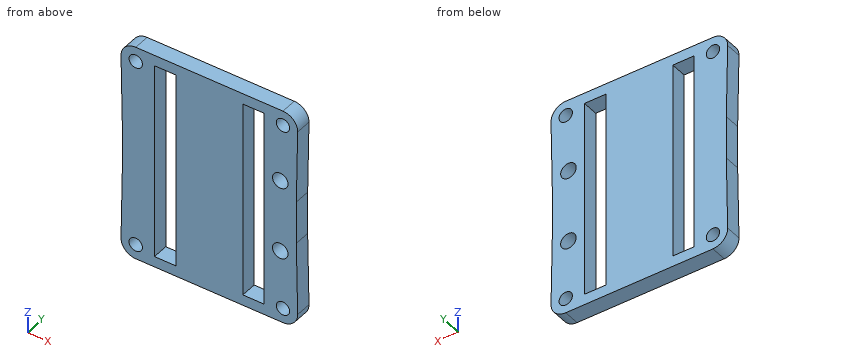
```python
from build123d import *

# Parameters (mm, degrees)
SKETCH1_R              = 1.25
SKETCH1_W              = 12.5
SKETCH1_H              = 37
BOSS_EXTRUDE1_DEPTH    = 3
M2_5_CLEARANCE_HOLE1_D = 2.9


with BuildPart() as part:
    # Sketch1 → Boss-Extrude1 (new body)
    with BuildSketch(Plane(origin=(0, 0, 0), x_dir=(1, 0, 0), z_dir=(0, 1, 0))):
        with BuildLine():
            Line((-16.25, -4), (-16.499543908, -17.699917074))
            ThreePointArc((-16.499543908, -17.699917074), (-15.712170743, -19.676755298), (-13.75, -20.5))
            Line((-13.75, -20.5), (13.75, -20.5))
            ThreePointArc((13.75, -20.5), (15.712170743, -19.676755298), (16.499543908, -17.699917074))
            Line((16.499543908, -17.699917074), (16.25, -4))
            Line((16.25, -4), (16.25, 0))
            Line((16.25, 0), (16.25, 4))
            Line((16.25, 4), (16.499543908, 17.699917074))
            ThreePointArc((16.499543908, 17.699917074), (15.712170743, 19.676755298), (13.75, 20.5))
            Line((13.75, 20.5), (-13.75, 20.5))
            ThreePointArc((-13.75, 20.5), (-15.712170743, 19.676755298), (-16.499543908, 17.699917074))
            Line((-16.499543908, 17.699917074), (-16.25, 4))
            Line((-16.25, 4), (-16.25, 0))
            Line((-16.25, 0), (-16.25, -4))
        make_face()
        with Locations((-13.75, -17.75)):
            Circle(SKETCH1_R, mode=Mode.SUBTRACT)
        with Locations((-13.75, 17.75)):
            Circle(SKETCH1_R, mode=Mode.SUBTRACT)
        with Locations((13.75, 17.75)):
            Circle(SKETCH1_R, mode=Mode.SUBTRACT)
        with Locations((13.75, -17.75)):
            Circle(SKETCH1_R, mode=Mode.SUBTRACT)
        Polygon((-6.25, 18.5), (-10.25, 18.5), (-10.25, -18.5), (-6.25, -18.5), (6.25, -18.5), (10.25, -18.5), (10.25, 18.5), (6.25, 18.5), align=None, mode=Mode.SUBTRACT)
        Rectangle(SKETCH1_W, SKETCH1_H)
    extrude(amount=BOSS_EXTRUDE1_DEPTH)

    # M2.5 Clearance Hole1 (through all)
    with Locations(Plane.XZ):
        with Locations((13.25, -6.8), (13.25, 6.8)):
            Hole(M2_5_CLEARANCE_HOLE1_D / 2)


solid = part.part
```
Verification items for the finished model (mm, model axes). Coordinates: 2 decimals unless noted, no trailing zeros. Order: outer loops, then holes, each group sorted by start corner. A loop starts at its lowest first (then second) coordinate and runs counter-clockwise, first axis right, second up. Notation, with made-up numbers: (57.25, 46.25) - (65.25, 46.25) arc R22 cw to (65.25, 61.25) - close; hole circle Ø8 at (76, -29). An arc over 180 degrees is marked (long way). Return JSON: item names as keys, results as strings.
(1) Section check C-C, the plane y = 1. Give the number of separate pieces and of enclosed holes in the cut face, and give its area (3 significant figures).
Filled sheet:
{"separate pieces": "1", "enclosed holes": "8", "area": "1,010 mm^2"}
(2) Section check D-D, the plane z = 6.8. Record the cut outline in (x, y).
Filled sheet:
{"outline": "(-16.3, 0) - (-10.25, 0) - (-10.25, 3) - (-16.3, 3) - close; (-6.25, 0) - (6.25, 0) - (6.25, 3) - (-6.25, 3) - close; (10.25, 0) - (11.8, 0) - (11.8, 3) - (10.25, 3) - close; (14.7, 0) - (16.3, 0) - (16.3, 3) - (14.7, 3) - close"}
(3) Section check B-B, the plane z = -1. Record the cut outline in (x, y), and give its area (3 significant figures).
Filled sheet:
{"outline": "(-16.25, 0) - (-10.25, 0) - (-10.25, 3) - (-16.25, 3) - close; (-6.25, 0) - (6.25, 0) - (6.25, 3) - (-6.25, 3) - close; (10.25, 0) - (16.25, 0) - (16.25, 3) - (10.25, 3) - close", "area": "73.5 mm^2"}
(4) Thickness scan on line 1 along X through (y, z) = (0.75, -4); line 2 along Z through (x, y) = (-13.75, 0.7); line 3 along X through (y, z) = (2.2, -17.75). Record the ranges inside material, lowest first.
Filled sheet:
{"line 1": "x = -16.25 to -10.25, -6.25 to 6.25, 10.25 to 16.25", "line 2": "z = -20.5 to -19, -16.5 to 16.5, 19 to 20.5", "line 3": "x = -16.5 to -15, -12.5 to -10.25, -6.25 to 6.25, 10.25 to 12.5, 15 to 16.5"}
(5) Section check A-A, the plane x = 9. Record the cut outline in (y, z), and give its area (3 significant figures).
Filled sheet:
{"outline": "(0, -20.5) - (3, -20.5) - (3, -18.5) - (0, -18.5) - close; (0, 18.5) - (3, 18.5) - (3, 20.5) - (0, 20.5) - close", "area": "12.0 mm^2"}
(6) Go/stop test with flat-tipped pins: pin 1 (0.9 mm diameter, centred on y = 1, z = 0, fed in from -X); pin 2 (0.9 mm diameter, centred on y = 1.5, z = -5, fed in from -X); pin 3 (3 mm diameter, centred on x = 13.75, z = -17.75, fed in from -Y); pin 4 (1.5 mm diameter, centred on y = 1, z = -1.5, fed in from +X). Record where each tip stops, or that it passes through.
Filled sheet:
{"pin 1": "stops at x = -16.25", "pin 2": "stops at x = -16.28", "pin 3": "stops at y = 0", "pin 4": "stops at x = 16.25"}
